Verification items for the finished model (mm, model axes). A direction names the side the tool comes from. Give positions to 0.01 mm unless a question says otherwise; leave off trailing zeros. Loops run counter-clockwise (first coordinate to the right, second up) from the corner with the lowest first, then second, coordinate; pieces in that order, holes last. Notation, with made-up numbers: M -1.75,-4 L 3.25,-4 A19 cw 3.25,1 Z; hole C 32,81 d5. An arc over 180 degrees is marked long. Use CSV: the item, a comma, the result in double quotes.
from build123d import *

# Parameters (mm, degrees)
SKETCH_W      = 28.575
SKETCH_H      = 38.1
SKETCH_R      = 1.9304
PAD_DEPTH     = 1.5875
SKETCH001_W   = 19.05
SKETCH001_H   = 8.128
PAD001_DEPTH  = 12.7
PAD001_TAPER  = 5
SKETCH002_W   = 5.9944
SKETCH002_H   = 14.478
PAD002_DEPTH  = 5.08
SKETCH003_R   = 2.5019
SKETCH003_R_2 = 1.7399
PAD003_DEPTH  = 2.4892
SKETCH004_W   = 9.652
SKETCH004_H   = 8.7884
PAD004_DEPTH  = 3.7846
SKETCH005_R   = 4.826
PAD005_DEPTH  = 21.7932


with BuildPart() as part:
    # Sketch → Pad (new body)
    with BuildSketch(Plane.XY):
        with Locations((15.5575, 19.05)):
            Rectangle(SKETCH_W, SKETCH_H)
        with Locations((6.35, 22.225)):
            Circle(SKETCH_R, mode=Mode.SUBTRACT)
    extrude(amount=-PAD_DEPTH)

    # Sketch001 (on Face6 of Pad) → Pad001 (join)
    with BuildSketch(Plane.XY):
        with Locations((15.875, 32.385)):
            Rectangle(SKETCH001_W, SKETCH001_H)
    extrude(amount=PAD001_DEPTH, taper=PAD001_TAPER)

    # Sketch002 (on Face4 of Pad001) → Pad002 (join)
    with BuildSketch(Plane.XY):
        with Locations((6.35, 6.9088)):
            Rectangle(SKETCH002_W, SKETCH002_H)
    extrude(amount=PAD002_DEPTH)

    # Sketch003 (on Face16 of Pad002) → Pad003 (join)
    with BuildSketch(Plane.XZ.offset(0.3302)):
        with Locations((6.35, 2.54)):
            Circle(SKETCH003_R)
        with Locations((6.35, 2.54)):
            Circle(SKETCH003_R_2, mode=Mode.SUBTRACT)
    extrude(amount=PAD003_DEPTH)

    # Sketch004 (on Face4 of Pad003) → Pad004 (join)
    with BuildSketch(Plane.XY):
        with Locations((22.225, 4.064)):
            Rectangle(SKETCH004_W, SKETCH004_H)
    extrude(amount=PAD004_DEPTH)

    # Sketch005 (on Face10 of Pad004) → Pad005 (join)
    with BuildSketch(Plane(origin=(0, 8.4582, 0), x_dir=(-1, 0, 0), z_dir=(0, 1, 0))):
        with Locations((-22.225, 3.7846)):
            Circle(SKETCH005_R)
    extrude(amount=-PAD005_DEPTH)


with BuildPart() as part_1:
    # Body002 placement: moved
    add(part.part.moved(Location((1.27, 0.127, 0))))


solid = part_1.part
(1) Depth check by flat-ended pin: pin 1 Ø12 at (x, y) = (24, 26.5) entering from +Z; pin 2 Ø8.5 at (x, y) = (19.5, 16) entering from +Z; pin 3 Ø6.5 at (x, y) = (6, 10) entering from +Z; pin 4 Ø3 at (x, z) = (7.62, 2.54) entering from +Y. Enter the tip coordinate at first touch or a pass-through.
Calculated:
pin 1,"stops at z = 12.7"
pin 2,"stops at z = 0"
pin 3,"stops at z = 5.08"
pin 4,"stops at y = 36.48"
(2) Section check C-C on z = 6.75. Record the cut outline in (x, y).
Calculated:
outline,"M 8.21,29.04 L 26.08,29.04 L 26.08,35.99 L 8.21,35.99 Z; M 19.69,-13.21 L 27.3,-13.21 L 27.3,8.59 L 19.69,8.59 Z"
(3) Section check A-A on y = 4. Record the cut outline in (x, z) (1 decimal), plus the area to 3 significant figures.
Calculated:
outline,"M 2.5,-1.6 L 31.1,-1.6 L 31.1,0 L 28.3,0 L 28.3,3.8 A4.8 ccw 18.7,3.8 L 18.7,0 L 10.6,0 L 10.6,5.1 L 4.6,5.1 L 4.6,0 L 2.5,0 Z"
area,"149 mm²"
(4) Section check B-B on z = 2.54. Record the cut outline in (x, y), plus the area to 3 significant figures.
Calculated:
outline,"M 4.62,-0.2 L 5.12,-0.2 L 5.12,-2.69 L 5.88,-2.69 L 5.88,-0.2 L 9.36,-0.2 L 9.36,-2.69 L 10.12,-2.69 L 10.12,-0.2 L 10.62,-0.2 L 10.62,14.27 L 4.62,14.27 Z; M 7.84,28.67 L 26.45,28.67 L 26.45,36.35 L 7.84,36.35 Z; M 18.67,-0.2 L 18.83,-0.2 L 18.83,-13.21 L 28.16,-13.21 L 28.16,-0.2 L 28.32,-0.2 L 28.32,8.59 L 18.67,8.59 Z"
area,"440 mm²"
(5) Scan lines: L1, parallel to Z at x = 7.62, y = -0.9; L2, parallel to X at y = 2, z = 2; L3, parallel to Z at x = 25, y = 17. Record each from-to range of solid material in increasing order. Write a range as from..to.
Calculated:
L1,"z = 0.04..0.8, 4.28..5.04"
L2,"x = 4.62..10.62, 18.67..28.32"
L3,"z = -1.59..0"
(6) Tool access check on faces 5 (the flat face through (9, -2.692, 1)), 6 (the flat face through (8, 14.275, 3)), 7 (the flat face through (28.321, 4, 2)), 8 (the flat face through (4.623, 7, 3)). Record the directions out of +Z, -Z, +X, -X, +Y, -Y that give a thin tool (end or side, any length) a straight path to the whole face; none if there is none.
Calculated:
face 5,"+Z, -Z, -X, -Y"
face 6,"+Z, +X, -X"
face 7,"+Z, +X, +Y, -Y"
face 8,"+Z, -X, +Y, -Y"
(7) Mould release check, pull along Y, two halves, no side actions. Record for faces 1 (the cylindrical face through (6.34, -1.43, 3.72)), 2 (the flat face through (28, -0.203, 1)), 3 (the flat face through (17, 19, 0)), 4 (the flat face through (17.01, 36.03, 6.26)): released by +Y, released by -Y, zero draft, split by the parting line, or undercut.
Calculated:
face 1,"zero draft"
face 2,"released by -Y"
face 3,"undercut"
face 4,"released by +Y"
(8) Section check D-D on y = 32. Record the cut outline in (x, z) (1 decimal), plus the area to 3 significant figures.
Calculated:
outline,"M 2.5,-1.6 L 31.1,-1.6 L 31.1,0 L 26.7,0 L 25.6,12.7 L 8.7,12.7 L 7.6,0 L 2.5,0 Z"
area,"273 mm²"
